The listing builds one solid part. Answer for the finished solid, in the listing's coordinates (mm). Round coordinates to 2 decimals unless told otherwise and drop trailing zeros. Write each loop counter-clockwise with the first axis right and the second up, starting at its lowest first coordinate (ties: lowest second). Pieces come first, ordered by that corner, then holes. Notation, with made-up numbers: (-37, 67) - (-27, 67) arc R25 cw to (-27, 92) - close; hole circle Ø1 at (-34, 84). An arc over 180 degrees is marked (long way). Return JSON: item names as keys, results as strings. Group by question number.
(1) Section A-A, the plane z = -14.75 is taken. Write down the section's boundary in (x, y).
(2) Each of these flat-tipped pins is pushed along its axis until it touches: pin 1 (0.5 mm diameter, centred on x = 22, z = -27, fed in from -Y); pin 2 (0.8 mm diameter, centred on x = 22, z = -27, fed in from +Y); pin 3 (1.5 mm diameter, centred on y = -69.5, z = -22, fed in from -X). Where does it stop, or does it pass through?
(3) Section B-B, the plane z = -17.5 is taken. Write down the section's boundary in (x, y), then the cut area to 3 significant figures.
(4) Find the intervals of material crossed by line 1 along Z through (x, y) = (22.1, -66.65); line 2 along Y through (x, z) = (22.9, -26.75); line 3 along Z through (x, y) = (21.2, -67.7), in increasing order. Write a range as [from, to].
(5) Determine the mould class of faces 1 (the flat face through (23.4, -67.6, -27.5)), 2 (the flat face through (22.8, -67.5, -27.2)), 3 (the conical face through (23.304, -67.415, -19.206)) for opening direction X: +X half, -X half, draft (parallel to the pull), parting line (faces both ways), or undercut.
```python
from build123d import *

# Parameters (mm, degrees)
POCKET002_DEPTH         = 0.2
POLARPATTERN001_COUNT   = 2
POLARPATTERN001_ANGLE   = 90
BODY008_PLACEMENT_ANGLE = 180


with BuildPart() as part:
    # Sketch026 → Revolution005 (revolve)
    with BuildSketch(Plane.XZ):
        Polygon((0, 0), (0, -16), (1.3, -0.8), (2, -0.1), (2, 0), align=None)
    revolve(axis=Axis((0, 0, 0), (0, 0, 1)))

    # Sketch027 → Pocket002 (cut, symmetric)
    with BuildSketch(Plane.XZ):
        Polygon((-1.15, 0), (0, -1.15), (1.15, 0), align=None)
    pocket002 = extrude(amount=POCKET002_DEPTH, both=True, mode=Mode.SUBTRACT)

    # PolarPattern001: Pocket002 ×2 about axis
    polarpattern001_axis = Axis((0, 0, 0), (0, 0, 1))
    for i in range(1, POLARPATTERN001_COUNT):
        add(pocket002.rotate(polarpattern001_axis, i * POLARPATTERN001_ANGLE / (POLARPATTERN001_COUNT - 1)), mode=Mode.SUBTRACT)


with BuildPart() as part_1:
    # Body008 placement: moved
    add(part.part.moved(Location((23, -68, -27.5))).rotate(Axis((23, -68, -27.5), (1, 0, 0)), BODY008_PLACEMENT_ANGLE))


solid = part_1.part
```
Working result:
{
 "1": {"outline": "circle Ø0.56 at (23, -68)"},
 "2": {"pin 1": "stops at y = -69.59", "pin 2": "stops at y = -66.22", "pin 3": "stops at x = 22.5"},
 "3": {"outline": "circle Ø1.03 at (23, -68)", "area": "0.827 mm^2"},
 "4": {"line 1": "z = [-27.5, -27.02]", "line 2": "y = [-69.35, -68.4], [-67.6, -66.65]", "line 3": "z = [-27.5, -27.22]"},
 "5": {"face 1": "draft", "face 2": "undercut", "face 3": "parting line"}
}
